Input: part model. Units: mm. Frame: model coordinates. Face numbers are marked on the shaded views. A direction names the side the tool comes from. Give positions to 0.01 mm unless a question says otherwise; leave off trailing zeros. Loops run counter-clockwise (first coordinate to the right, second up) from the corner with the lowest first, then second, coordinate; pieces in that order, holes last. Notation, with made-up numbers: (-36.5, 33.5) - (-17.5, 33.5) arc R28 ccw to (-17.5, 71.5) - close; hole circle Ø4 at (66, 11.25). An arc over 180 degrees is marked (long way). Answer as a JSON object with one key per item and string values.
from build123d import *

# Parameters (mm, degrees)
SKETCH1_R                       = 15
BOSS_EXTRUDE1_DEPTH             = 35.5
SKETCH2_R                       = 14.2
CUT_EXTRUDE1_DEPTH              = 31.5
SKETCH3_R                       = 7.5
CUT_EXTRUDE2_DEPTH              = 42.355168964
M3X0_5_TAPPED_HOLE1_D           = 2.5
M3X0_5_TAPPED_HOLE1_CSINK_D     = 3.2
M3X0_5_TAPPED_HOLE1_CSINK_ANGLE = 90
CIRPATTERN2_COUNT               = 4
BOSS_EXTRUDE2_START             = 3
SKETCH8_R                       = 10
SKETCH8_R_2                     = 7.5
BOSS_EXTRUDE2_DEPTH             = 3


with BuildPart() as part:
    # Sketch1 → Boss-Extrude1 (new body)
    with BuildSketch(Plane.XY):
        Circle(SKETCH1_R)
    extrude(amount=-BOSS_EXTRUDE1_DEPTH)

    # Sketch2 → Cut-Extrude1 (cut)
    with BuildSketch(Plane.XY.offset(-35.5)):
        Circle(SKETCH2_R)
    extrude(amount=CUT_EXTRUDE1_DEPTH, mode=Mode.SUBTRACT)

    # Sketch3 → Cut-Extrude2 (cut, through all)
    with BuildSketch(Plane(origin=(0, 0, 0), x_dir=(-1, 0, 0), z_dir=(0, 0, -1))):
        with Locations(Location((0, 0, 0), (0, 0, 180))):
            Circle(SKETCH3_R)
    extrude(amount=CUT_EXTRUDE2_DEPTH, mode=Mode.SUBTRACT)

    # M3x0.5 Tapped Hole1 (through all)
    with Locations(Plane(origin=(0, 0, 0), x_dir=(-1, 0, 0), z_dir=(0, 0, 1))):
        with Locations((-13, 0)):
            m3x0_5_tapped_hole1 = CounterSinkHole(M3X0_5_TAPPED_HOLE1_D / 2, M3X0_5_TAPPED_HOLE1_CSINK_D / 2, counter_sink_angle=M3X0_5_TAPPED_HOLE1_CSINK_ANGLE)

    # CirPattern2: M3x0.5 Tapped Hole1 ×4 about axis
    cirpattern2_axis = Axis((0, 0, 0), (0, 0, 1))
    for i in range(1, CIRPATTERN2_COUNT):
        add(m3x0_5_tapped_hole1.rotate(cirpattern2_axis, i * 360 / CIRPATTERN2_COUNT), mode=Mode.SUBTRACT)

    # Sketch8 → Boss-Extrude2 (add)
    with BuildSketch(Plane.XY.offset(BOSS_EXTRUDE2_START)):
        Circle(SKETCH8_R)
        Circle(SKETCH8_R_2, mode=Mode.SUBTRACT)
    extrude(amount=-BOSS_EXTRUDE2_DEPTH)


solid = part.part
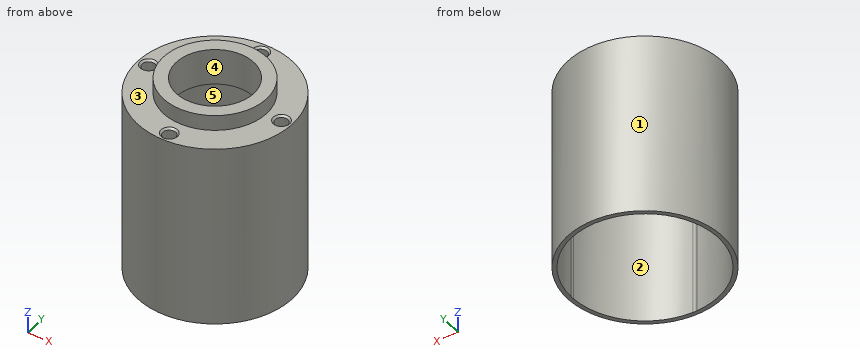
Item 1: Cut plane B-B (x = 13). Return loops of the section in (y, z), then the cut area to 3 significant figures.
Geometry check:
{"outline": "(-7.48, -35.5) - (-5.71, -35.5) - (-5.71, -4) - (-1.25, -4) - (-1.25, -0.35) - (-1.6, 0) - (-7.48, 0) - close; (1.25, -4) - (5.71, -4) - (5.71, -35.5) - (7.48, -35.5) - (7.48, 0) - (1.6, 0) - (1.25, -0.35) - close", "area": "161 mm2"}
Item 2: Contact query for flat-ended pins moving along their axis: P1, Ø2, axis at x = 13, y = 0, coming from the +Z side; P2, Ø3, axis at x = 6, y = 1.5, coming from the -Z side; P3, Ø12, axis at x = -8.5, y = -7.5, coming from the -Z side; P4, Ø5, axis at x = 7, z = -25.5, coming from the -Y side. Output: stop coordinate, or through.
Geometry check:
{"P1": "passes through", "P2": "stops at z = -4", "P3": "stops at z = -35.5", "P4": "stops at y = -14.31"}
Item 3: Cut plane A-A (z = -26). Return loops of the section in (x, y).
Geometry check:
{"outline": "circle Ø30 at (0, 0); hole (-14.2, -0.37) arc R14.2 ccw to (-0.37, -14.2) arc R1.25 ccw to (0.37, -14.2) arc R14.2 ccw to (14.2, -0.37) arc R1.25 ccw to (14.2, 0.37) arc R14.2 ccw to (0.37, 14.2) arc R1.25 ccw to (-0.37, 14.2) arc R14.2 ccw to (-14.2, 0.37) arc R1.25 ccw to start"}
Item 4: Material intervals for line 1 (Z direction, x = 6, y = -11.25); line 2 (Z direction, x = 8.5, y = -2); line 3 (Y direction, x = -2.75, z = -15.5), sorted ascending. Write a range as [from, to].
Geometry check:
{"line 1": "z = [-4, 0]", "line 2": "z = [-4, 3]", "line 3": "y = [-14.75, -13.93], [13.93, 14.75]"}
Item 5: Cut plane C-C (y = 6.5). Return loops of the section in (x, z), then the cut area to 3 significant figures.
Geometry check:
{"outline": "(-13.52, -35.5) - (-12.62, -35.5) - (-12.62, -4) - (-3.74, -4) - (-3.74, 3) - (-7.6, 3) - (-7.6, 0) - (-13.52, 0) - close; (3.74, -4) - (12.62, -4) - (12.62, -35.5) - (13.52, -35.5) - (13.52, 0) - (7.6, 0) - (7.6, 3) - (3.74, 3) - close", "area": "158 mm2"}
Item 6: Access query for the marked faces 4 and 5. Directions: +Z, -Z, +X, -X, +Y, -Y. A direction counts if a zero-diameter tool reaches every point of the face in a straight line with its end or side. Return the directions, or none.
Geometry check:
{"face 4": "+Z, -Z", "face 5": "-Z"}
Item 7: Cut plane D-D (x = -9). Return loops of the section in (y, z), then the cut area to 3 significant figures.
Geometry check:
{"outline": "(-12, -35.5) - (-10.98, -35.5) - (-10.98, -4) - (10.98, -4) - (10.98, -35.5) - (12, -35.5) - (12, 0) - (4.36, 0) - (4.36, 3) - (-4.36, 3) - (-4.36, 0) - (-12, 0) - close", "area": "186 mm2"}
Item 8: Mould query, pull axis X, two halves, no side actions, for the marked faces 1, 2 and 3. Classes: released by +X, released by -X, zero draft, split by the parting line, or undercut.
Geometry check:
{"face 1": "split by the parting line", "face 2": "undercut", "face 3": "zero draft"}
